Autodesk Inventor part; units mm, degrees
sketch "Эскиз2" plane through (0, 0, 0) normal (0, 0, 1) x (1, 0, 0)
  line L0 (-34.5, -42) -> (34.5, -42)
  line L1 (34.5, -42) -> (34.5, 42)
  line L2 (34.5, 42) -> (-34.5, 42)
  line L3 (-34.5, 42) -> (-34.5, -42)
  line L4 (-34.5, -42) -> (34.5, 42) construction
  line L5 (34.5, -42) -> (-34.5, 42) construction
  line L6 (-34.5, -42) -> (50.5, -42)
  line L7 (50.5, -42) -> (50.5, -55)
  line L8 (50.5, -55) -> (-34.5, -55)
  line L9 (-34.5, -55) -> (-34.5, -42)
  circle A0 centre (15.5, -5) radius 50
  line L10 (60.5, -42) -> (60.5, -55)
  line L11 (50.5, -42) -> (60.5, -42)
  line L12 (50.5, -55) -> (50.5, -42)
  line L13 (60.5, -55) -> (50.5, -55)
  line L14 (50.5, -55) -> (60.5, -42) construction
  line L15 (50.5, -42) -> (60.5, -55) construction
  circle A1 centre (55.5, -48.5) radius 2
  circle A2 centre (55.5, -48.5) radius 2.8
  point P0 (0, 0)
  point P1 (34.5, -42)
  point P2 (-34.5, -37)
  point P3 (15.5, -55)
  point P4 (-18.1303, -42)
  point P5 (50.5, -42.7071)
  point P6 (-34.5, -5)
  point P7 (-1.5587, 42)
  point P8 (34.5, 41.2493)
  dimension "d15" = 100
  dimension "d27" = 4
  dimension "d35" = 69
extrude "Выдавливание2" add sketch "Эскиз2" along normal mid plane 4 contours A0 L2 L1 L0 | L0 L6 A0 | L3 L2 A0 | A0 L6 L7 L8 | A0 L2 L1 | L7 L11 L10 L13 | A2
sketch "Эскиз3" plane through (0, 0, 2) normal (0, 0, 1) x (1, 0, 0)
  line L0 (34.5, 42) -> (-34.5, 42)
  line L1 (-14.5, 42) -> (-4.5, 42)
  line L2 (-4.5, 42) -> (-4.5, 38)
  line L3 (-4.5, 38) -> (-14.5, 38)
  line L4 (-14.5, 38) -> (-14.5, 42)
  line L5 (14.5, 42) -> (24.5, 42)
  line L6 (24.5, 42) -> (24.5, 38)
  line L7 (24.5, 38) -> (14.5, 38)
  line L8 (14.5, 38) -> (14.5, 42)
  line L9 (-34.5, 42) -> (-34.5, -5)
  line L10 (34.5, -42) -> (34.5, 42)
  point P0 (0, 0)
  point P1 (-34.5, -37)
  point P2 (-14.5, 40)
  point P3 (24.5, 42)
  point P4 (-4.5, 42)
  point P5 (-34.5, -69)
  dimension "d16" = 10
  dimension "d17" = 4
  dimension "d18" = 20
  dimension "d19" = 10
extrude "Выдавливание3" cut sketch "Эскиз3" against normal up to next
fillet "Сопряжение1" radius 10 1 edges at (34.5, -42, 0)
sketch "Эскиз6" plane through (0, 0, 2) normal (0, 0, 1) x (1, 0, 0)
  line L0 (-25.95, 38) -> (-25.95, 42)
  line L1 (-23.05, 42) -> (-23.05, 38)
  line L2 (3.55, 38) -> (3.55, 42)
  line L3 (6.45, 42) -> (6.45, 38)
  line L4 (-25.95, 40) -> (-23.05, 40) construction
  line L5 (3.55, 40) -> (6.45, 40) construction
  circle A0 centre (-24.5, 40) radius 1.5
  circle A1 centre (5, 40) radius 1.5
  point P0 (0, 0)
  point P1 (6.45, 40.3841)
  point P2 (3.55, 40.3841)
  point P3 (3.55, 39.6159)
  point P4 (6.45, 39.6159)
  point P5 (-23.05, 40.3841)
  point P6 (-25.95, 40.3841)
  point P7 (-25.95, 39.6159)
  point P8 (-23.05, 39.6159)
  dimension "d28" = 3
extrude "Выдавливание6" cut sketch "Эскиз6" against normal up to next contours L0 A0 L1 | L2 A1 L3
sketch "Эскиз7" plane through (0, 0, -2) normal (0, 0, -1) x (-1, 0, 0)
  line L0 (0, -15) -> (0, 15) construction
  line L1 (10, -15) -> (10, 15)
  line L2 (-10, 15) -> (-10, -15)
  arc A0 (-10, -15) -> (10, -15) centre (0, -15) ccw
  arc A1 (10, 15) -> (-10, 15) centre (0, 15) ccw
  point P0 (0, 0)
  dimension "d31" = 10
  dimension "d32" = 30
extrude "Выдавливание7" cut sketch "Эскиз7" against normal up to next
properties part number "дополнительное_ребро_жёсткости"
Source: CAD feature listing. Evaluate the final solid. Frame: model axes, mm. A direction names the side the tool comes from. Give positions to 0.01 mm unless a question says otherwise; leave off trailing zeros. Write each loop counter-clockwise with the first axis right and the second up, starting at its lowest first coordinate (ties: lowest second). Pieces come first, ordered by that corner, then holes. Notation, with made-up numbers: M 15.25,-38.75 L 45.25,-38.75 A16 cw 45.25,-18.75 Z; hole C 13.5,25 d5. An arc over 180 degrees is marked long. Return JSON: item names as keys, results as strings. Group by question number.
1) Cut plane D-D, the plane y = 27. Output: boundary loops of the cut face in (x, z), plus the area to 3 significant figures.
2) Cut plane C-C, the plane x = 0. Output: boundary loops of the cut face in (y, z), plus the area to 3 significant figures.
3) Cut plane B-B, the plane y = -7.5. Output: boundary loops of the cut face in (x, z), plus the area to 3 significant figures.
4) Material intervals for line 1 along Y through (x, z) = (55.5, -0.05); line 2 along X through (y, z) = (0.5, -1.25); line 3 along Y through (x, z) = (19, -0.75), sorted ascending. Write a range as [from, to].
5) Cut plane A-A, the plane z = -0.35. Give the number of separate pieces and of enclosed holes in the cut face, plus the area to 3 significant figures.
6) Pull-direction query (Y, two-part tool) for faces 1 (the face through (5, 42, 0)), 2 (the face through (34.5, 4, 0)), 3 (the face through (-24.5, 38.5, 0)); classes: pulls with the +Y half, pulls with the -Y half, needs draft (parallel to the pull), parting line crosses it, or undercut.
7) Set-up query: faces 4 (the face through (-24.5, 41.5, 0)), 5 (the face through (52, -42, 0)), 6 (the face through (-14.5, 40, 0)), 7 (the face through (-34.5, 19, 0)), 8 (the face through (-19.464, -40.742, -0.028)). Return all of +Z, -Z, +X, -X, +Y, -Y with unobstructed straight access to the full face (end or side cutting, diameter ignored); none if empty.
8) Pin query (flat end, axial travel): P1, Ø2, axis at x = 21.5, z = 0.5, coming from the +Y side; P2, Ø2, axis at x = 52.5, z = 0.5, coming from the +Y side; P3, Ø1.5, axis at x = -18.5, z = 1.5, coming from the -Y side; P4, Ø3, axis at x = 55.5, y = -48.5, coming from the +Z side. Return the tip coordinate at first contact, or that it passes through.
Recorded:
{
 "1": {"outline": "M -34.5,-2 L 34.5,-2 L 34.5,2 L -34.5,2 Z", "area": "276 mm²"},
 "2": {"outline": "M -52.54,-2 L -25,-2 L -25,2 L -52.54,2 Z; M 25,-2 L 42,-2 L 42,2 L 25,2 Z", "area": "178 mm²"},
 "3": {"outline": "M -34.44,-2 L -10,-2 L -10,2 L -34.44,2 Z; M 10,-2 L 34.5,-2 L 34.5,2 L 10,2 Z", "area": "196 mm²"},
 "4": {"line 1": "y = [-55, -50.5], [-46.5, -42]", "line 2": "x = [-34.5, -10], [10, 34.5]", "line 3": "y = [-55, 38]"},
 "5": {"separate pieces": "1", "enclosed holes": "4", "area": "5,500 mm²"},
 "6": {"face 1": "pulls with the +Y half", "face 2": "needs draft", "face 3": "undercut"},
 "7": {"face 4": "+Z, -Z", "face 5": "+Z, -Z, +X, +Y", "face 6": "+Z, -Z, +Y", "face 7": "+Z, -Z, -X, +Y, -Y", "face 8": "+Z, -Z, -X, -Y"},
 "8": {"P1": "stops at y = 38", "P2": "stops at y = -42", "P3": "stops at y = -42.34", "P4": "passes through"}
}
